Can you work these out from the model? Positions are in its coordinate system, mm. Give positions to 0.01 mm unless a question says otherwise; leave off trailing zeros. Loops run counter-clockwise (first coordinate to the right, second up) from the corner with the lowest first, then second, coordinate; pieces in that order, holes last. Notation, with made-up numbers: (46, -39) - (92, -39) arc R11 ccw to (92, -34) - close; hole circle Ø6 at (-35.5, -32.5). An arc over 180 degrees is marked (long way). Answer as a JSON object with one key per item and string values. Group by question number.
Item 1: Will this pin go through, and if not, where does the flat tip stop? pin 1 (1 mm diameter, centred on x = 46.5, z = 2.5, fed in from +Y).
Item 2: Suppose I cut it at D-D on x = 97. Write out the boundary of the cut face in (y, z) (3 decimals).
Item 3: Suppose I cut it at C-C on y = -29. Write out the boundary of the cut face in (x, z) (3 decimals), and give its area (3 significant figures).
Item 4: Suppose I cut it at B-B on x = 47. Write out the boundary of the cut face in (y, z) (3 decimals), and give its area (3 significant figures).
Item 5: Please list where these lines run through material, in increasing order: L1, parallel to Y at x = 46.5, z = 0.4; L2, parallel to X at y = 6, z = 0.45; L3, parallel to Y at x = 35.5, z = 3.
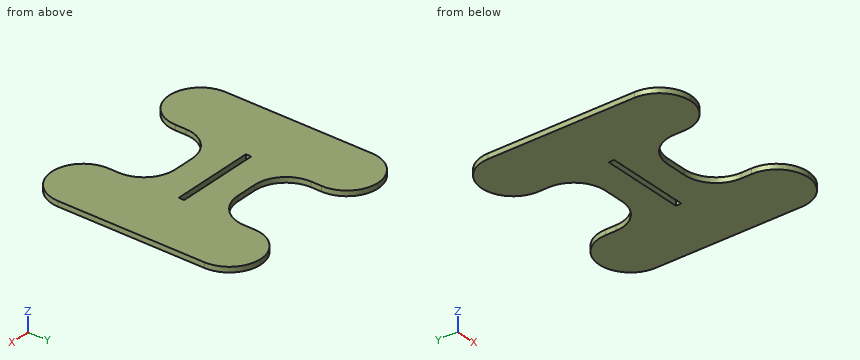
from build123d import *

# Parameters (mm, degrees)
F0_W     = 50.8
F0_H     = 3.302
F1_DEPTH = 3.175
F2_R     = 19.04999


# Not quite as in the source:
# - a fillet or chamfer is up to 0.001 mm smaller than in the source, because OpenCascade refuses the exact size


with BuildPart() as f1:
    # F0 (on Top) → F1 (new body)
    with BuildSketch(Plane.XY):
        Polygon((18.769003178, 68.6352171788), (-19.330996822, 68.6352171788), (-19.330996822, -58.3647828212), (18.769003178, -58.3647828212), (18.769003178, -13.9147828212), (69.569003178, -13.9147828212), (69.569003178, -58.3647828212), (107.669003178, -58.3647828212), (107.669003178, 68.6352171788), (69.569003178, 68.6352171788), (69.569003178, 24.1852171788), (18.769003178, 24.1852171788), align=None)
        with Locations((44.169003178, 5.1352171788)):
            Rectangle(F0_W, F0_H, mode=Mode.SUBTRACT)
    extrude(amount=F1_DEPTH)

    # F2 (radius 19.05 in the source; OpenCascade refuses exactly that, so slightly less here)
    f2_edges = [f1.edges().sort_by_distance(p)[0] for p in [
        (18.769003, -58.364783, 1.5875),
        (-19.330997, -58.364783, 1.5875),
        (69.569003, -58.364783, 1.5875),
        (107.669003, -58.364783, 1.5875),
        (18.769003, -13.914783, 1.5875),
        (69.569003, -13.914783, 1.5875),
        (-19.330997, 68.635217, 1.5875),
        (18.769003, 68.635217, 1.5875),
        (69.569003, 24.185217, 1.5875),
        (69.569003, 68.635217, 1.5875),
        (107.669003, 68.635217, 1.5875),
        (18.769003, 24.185217, 1.5875),
    ]]
    fillet(f2_edges, radius=F2_R)


solid = f1.part
Worked out:
{
 "1": {"pin 1": "stops at y = 24.19"},
 "2": {"outline": "(-56.422, 0) - (66.693, 0) - (66.693, 3.175) - (-56.422, 3.175) - close"},
 "3": {"outline": "(-19.331, 0) - (19.186, 0) - (19.186, 3.175) - (-19.331, 3.175) - close; (69.152, 0) - (107.669, 0) - (107.669, 3.175) - (69.152, 3.175) - close", "area": "245 mm2"},
 "4": {"outline": "(-13.915, 0) - (3.484, 0) - (3.484, 3.175) - (-13.915, 3.175) - close; (6.786, 0) - (24.185, 0) - (24.185, 3.175) - (6.786, 3.175) - close", "area": "110 mm2"},
 "5": {"L1": "y = -13.91 to 3.48, 6.79 to 24.19", "L2": "x = -19.33 to 18.77, 69.57 to 107.67", "L3": "y = -14.06 to 3.48, 6.79 to 24.33"}
}
